Verification items for this drawing (mm, ordinates from the low corner). Round coordinates to 2 decimals unless told otherwise and drop trailing zeros. Order: outer loops, then holes, each group sorted by start corner. A loop starts at its lowest first (then second) coordinate and runs counter-clockwise, first axis right, second up. Notation, with made-up numbers: (65, 32.5) -> (108, 32.5) arc R18 cw to (108, 38.5) -> close; hole circle Ø1 at (82, -39). An arc over 180 degrees is marked (long way). Answer in a Markdown table with one row per item. Add a question column.
1. Sectioned sample at A-A, the plane x = 405. Record the boundary of the cut face in (y, z) (3 decimals), then the cut area to 3 significant figures.
2. Material ranges on L1, parallel to Y at x = 447, z = 1106, recorded low to high. Write a range as from..to.
3. Depth check by flat-ended pin: P1, Ø7.5, axis at y = 16.5, z = 264, coming from the +X side; P2, Ø7.5, axis at x = 556, y = 11.5, coming from the -Z side; P3, Ø20.5, axis at x = 278.5, y = 11, coming from the +Z side (3 decimals). Enter the tip coordinate at first touch or a pass-through.
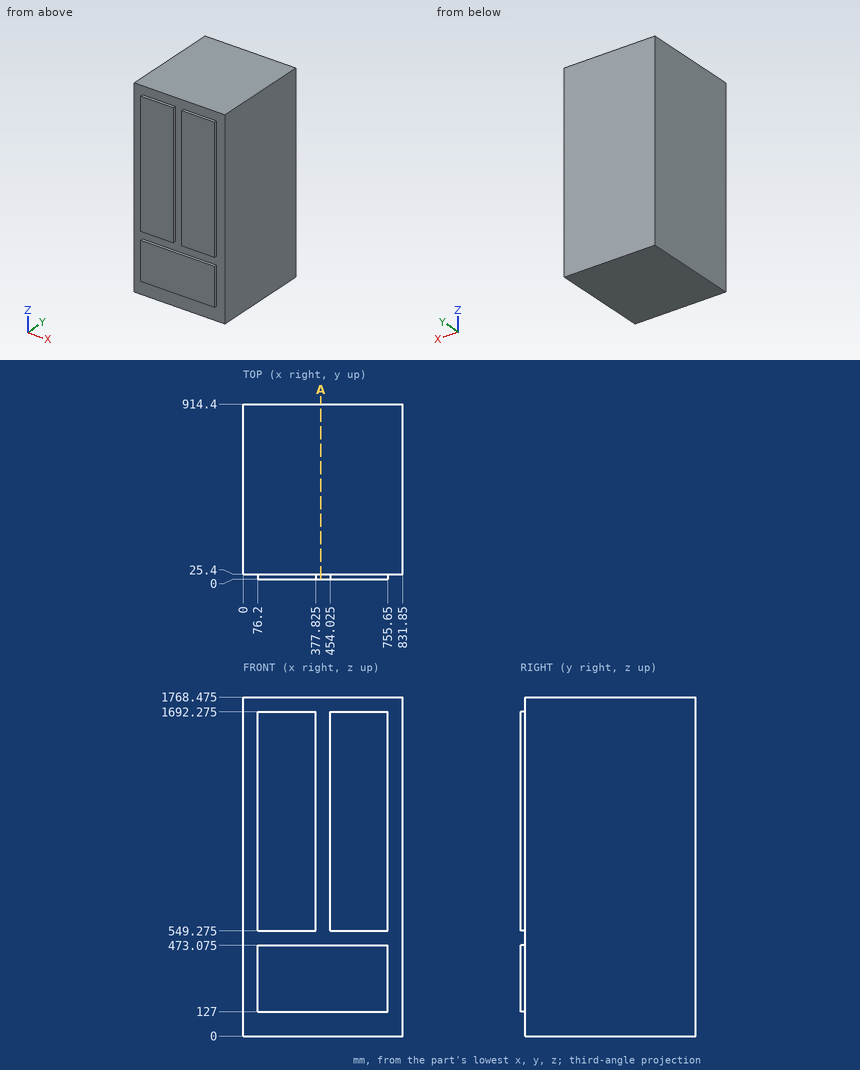
Answer key:
| question | item | result |
|---|---|---|
| 1 | outline | (0, 127) -> (25.4, 127) -> (25.4, 0) -> (914.4, 0) -> (914.4, 1768.475) -> (25.4, 1768.475) -> (25.4, 473.075) -> (0, 473.075) -> close |
| 1 | area | 1,580,000 mm² |
| 2 | L1 | y = 25.4..914.4 |
| 3 | P1 | stops at x = 755.65 |
| 3 | P2 | stops at z = 127 |
| 3 | P3 | stops at z = 1692.275 |
